Geometry check sheet. Reference: the model listing, model coordinates, mm. A direction names the side the tool comes from. Round coordinates to 2 decimals unless told otherwise and drop trailing zeros. Write each loop counter-clockwise with the first axis right and the second up, starting at its lowest first coordinate (ties: lowest second). Pieces come first, ordered by that corner, then holes.
Item 1: Access from +Z, -Z, +X, -X, +Y, -Y to the whole of each face (thin tool, end or side, straight path). Record for faces 1 (the face through (-9, 0, -73.025)), 2 (the face through (37, -19.05, 34)).
Item 2: Draft check along Z on faces 3 (the face through (-8, 0, 76.2)), 4 (the face through (34.925, 0, 1)), 5 (the face through (8, 0, -76.2)), 6 (the face through (37, 19.05, 34)). Enter one of: pulls with the +Z half, pulls with the -Z half, needs draft (parallel to the pull), parting line crosses it, or undercut.
Item 3: Cross-section at B-B (y = 0). Enter the section's corners in (x, z) (3 decimals), then the cut area to 3 significant figures.
Item 4: Scan lines: probe 1 along X at (y, z) = (0, -74.35); probe 2 along Z at (x, y) = (-10, -3.5) (3 decimals); probe 3 along Y at (x, z) = (0, -74.15). Record each from-to range of solid material in increasing order.
Item 5: Depth check by flat-ended pin: P1, Ø16.5, axis at x = 0, y = 0, coming from the +Z side. Enter the tip coordinate at first touch or a pass-through.
Item 6: Cross-section at D-D (y = -16). Enter the section's corners in (x, z) (3 decimals), then the cut area to 3 significant figures.
Item 7: Cross-section at A-A (x = 0). Enter the section's corners in (y, z) (3 decimals), then the cut area to 3 significant figures.
Item 8: Cross-section at C-C (x = -13). Enter the section's corners in (y, z) (3 decimals), then the cut area to 3 significant figures.
from build123d import *

# Parameters (mm, degrees)
F1_DEPTH = 19.05
F2_R     = 6.35
F3_DEPTH = 3.175
F4_R     = 6.35
F5_DEPTH = 3.175


with BuildPart() as f1:
    # F0 (on Front) → F1 (new body, symmetric)
    with BuildSketch(Plane.XZ):
        Polygon((38.1, 76.2), (-38.1, 76.2), (-38.1, 73.025), (34.925, 73.025), (34.925, -73.025), (-38.1, -73.025), (-38.1, -76.2), (38.1, -76.2), align=None)
    extrude(amount=F1_DEPTH, both=True)

    # F2 (on face) → F3 (cut, symmetric)
    with BuildSketch(Plane.XY.offset(76.2)):
        Circle(F2_R)
    extrude(amount=F3_DEPTH, both=True, mode=Mode.SUBTRACT)

    # F4 (on face) → F5 (cut, symmetric)
    with BuildSketch(Plane(origin=(0, 0, -76.2), x_dir=(1, 0, 0), z_dir=(0, 0, -1))):
        Circle(F4_R)
    extrude(amount=F5_DEPTH, both=True, mode=Mode.SUBTRACT)


solid = f1.part
Resolved:
1. face 1: -X, +Y, -Y
1. face 2: +Z, -Z, +X, -X, -Y
2. face 3: pulls with the +Z half
2. face 4: undercut
2. face 5: pulls with the -Z half
2. face 6: needs draft
3. outline: (-38.1, -76.2) - (-6.35, -76.2) - (-6.35, -73.025) - (-38.1, -73.025) - close; (-38.1, 73.025) - (-6.35, 73.025) - (-6.35, 76.2) - (-38.1, 76.2) - close; (6.35, -76.2) - (38.1, -76.2) - (38.1, 76.2) - (6.35, 76.2) - (6.35, 73.025) - (34.925, 73.025) - (34.925, -73.025) - (6.35, -73.025) - close
3. area: 867 mm2
4. probe 1: x = -38.1 to -6.35, 6.35 to 38.1
4. probe 2: z = -76.2 to -73.025, 73.025 to 76.2
4. probe 3: y = -19.05 to -6.35, 6.35 to 19.05
5. P1: stops at z = 76.2
6. outline: (-38.1, -76.2) - (38.1, -76.2) - (38.1, 76.2) - (-38.1, 76.2) - (-38.1, 73.025) - (34.925, 73.025) - (34.925, -73.025) - (-38.1, -73.025) - close
6. area: 948 mm2
7. outline: (-19.05, -76.2) - (-6.35, -76.2) - (-6.35, -73.025) - (-19.05, -73.025) - close; (-19.05, 73.025) - (-6.35, 73.025) - (-6.35, 76.2) - (-19.05, 76.2) - close; (6.35, -76.2) - (19.05, -76.2) - (19.05, -73.025) - (6.35, -73.025) - close; (6.35, 73.025) - (19.05, 73.025) - (19.05, 76.2) - (6.35, 76.2) - close
7. area: 161 mm2
8. outline: (-19.05, -76.2) - (19.05, -76.2) - (19.05, -73.025) - (-19.05, -73.025) - close; (-19.05, 73.025) - (19.05, 73.025) - (19.05, 76.2) - (-19.05, 76.2) - close
8. area: 242 mm2
